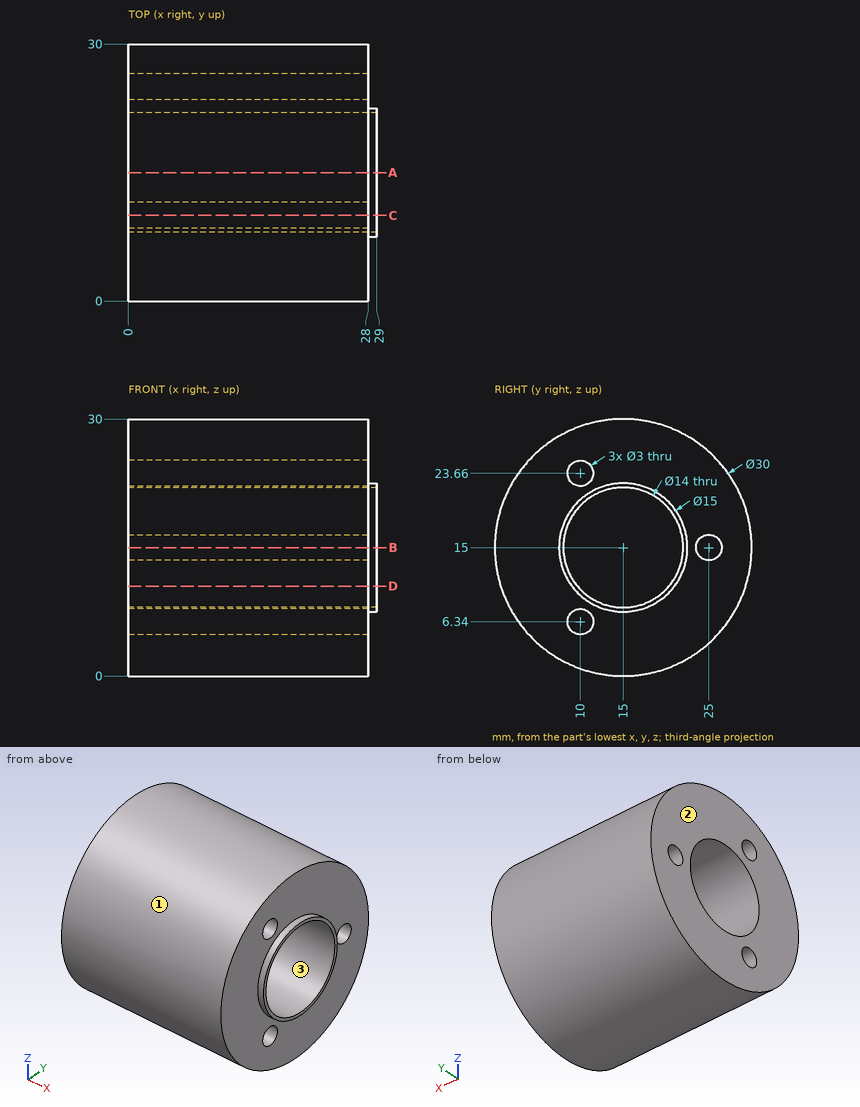
Check sheet for the drawn part. Datum: minimum x, y, z corner. Units: mm. Coordinates: 2 decimals unless noted, no trailing zeros. Write each loop counter-clockwise with the first axis right and the second up, starting at its lowest first coordinate (ties: lowest second). Pieces come first, ordered by that corner, then holes. Notation, with made-up numbers: (-38, -35) - (15, -35) arc R14 ccw to (15, -23) - close; hole circle Ø6 at (27, 44). An arc over 180 degrees is marked (long way). Answer as a JSON object with one key per item and string values.
(1) Cross-section at A-A on y = 15. Record the cut outline in (x, z), plus the area to 3 significant figures.
Report:
{"outline": "(0, 0) - (28, 0) - (28, 7.5) - (29, 7.5) - (29, 8) - (0, 8) - close; (0, 22) - (29, 22) - (29, 22.5) - (28, 22.5) - (28, 30) - (0, 30) - close", "area": "449 mm^2"}
(2) Gauge pin test, flat ends, axial feed: pin 1 Ø12 at (x, y) = (15.5, 22.5) entering from +Z (1 decimal); pin 2 Ø3 at (x, z) = (9.5, 7.5) entering from -Y; pin 3 Ø5 at (x, z) = (12, 22.5) entering from -Y. Record the tip position at first contact, or that the pin passes through.
Report:
{"pin 1": "z = 29.9", "pin 2": "y = 1.25", "pin 3": "y = 0.86"}
(3) Thickness scan on line 1 along Y through (x, z) = (10.75, 15); line 2 along Z through (x, y) = (16, 10); line 3 along X through (y, z) = (28.5, 12). Record the ranges inside material, lowest first.
Report:
{"line 1": "0 to 8, 22 to 23.5, 26.5 to 30", "line 2": "0.86 to 4.84, 7.84 to 10.1, 19.9 to 22.16, 25.16 to 29.14", "line 3": "0 to 28"}
(4) Mould release check, pull along Z, two halves, no side actions. Record for the marked faces 1, 2 and 3: pulls with the +Z half, pulls with the -Z half, needs draft (parallel to the pull), parting line crosses it, or undercut.
Report:
{"face 1": "parting line crosses it", "face 2": "needs draft", "face 3": "undercut"}
(5) Cross-section at D-D on z = 10.5. Record the cut outline in (x, y), plus the area to 3 significant figures.
Report:
{"outline": "(0, 0.69) - (28, 0.69) - (28, 9) - (29, 9) - (29, 9.64) - (0, 9.64) - close; (0, 20.36) - (29, 20.36) - (29, 21) - (28, 21) - (28, 29.31) - (0, 29.31) - close", "area": "502 mm^2"}
(6) Cross-section at C-C on y = 10. Record the cut outline in (x, z), plus the area to 3 significant figures.
Report:
{"outline": "(0, 0.86) - (28, 0.86) - (28, 4.84) - (0, 4.84) - close; (0, 7.84) - (28, 7.84) - (28, 9.41) - (29, 9.41) - (29, 10.1) - (0, 10.1) - close; (0, 19.9) - (29, 19.9) - (29, 20.59) - (28, 20.59) - (28, 22.16) - (0, 22.16) - close; (0, 25.16) - (28, 25.16) - (28, 29.14) - (0, 29.14) - close", "area": "351 mm^2"}
(7) Cross-section at B-B on z = 15. Record the cut outline in (x, y).
Report:
{"outline": "(0, 0) - (28, 0) - (28, 7.5) - (29, 7.5) - (29, 8) - (0, 8) - close; (0, 22) - (29, 22) - (29, 22.5) - (28, 22.5) - (28, 23.5) - (0, 23.5) - close; (0, 26.5) - (28, 26.5) - (28, 30) - (0, 30) - close"}
